from build123d import *

# Parameters (mm, degrees)
SKETCH1_W           = 19
SKETCH1_H           = 22
BOSS_EXTRUDE1_DEPTH = 22
SKETCH2_R           = 3.175
CUT_EXTRUDE1_DEPTH  = 22
SKETCH3_R           = 7.5
CUT_EXTRUDE2_DEPTH  = 5.5
SKETCH4_W           = 2
SKETCH4_H           = 3
CUT_EXTRUDE5_DEPTH  = 11


with BuildPart() as part:
    # Sketch1 → Boss-Extrude1 (new body)
    with BuildSketch(Plane(origin=(0, 0, 0), x_dir=(1, 0, 0), z_dir=(0, 1, 0))):
        Rectangle(SKETCH1_W, SKETCH1_H)
    extrude(amount=-BOSS_EXTRUDE1_DEPTH)

    # Sketch2 → Cut-Extrude1 (cut)
    with BuildSketch(Plane(origin=(0, 0, 0), x_dir=(1, 0, 0), z_dir=(0, 1, 0))):
        with Locations(Location((0, 0, 0), (0, 0, 270))):
            Circle(SKETCH2_R)
    extrude(amount=-CUT_EXTRUDE1_DEPTH, mode=Mode.SUBTRACT)

    # Sketch3 → Cut-Extrude2 (cut)
    with BuildSketch(Plane.XZ.offset(22)):
        with Locations(Location((0, 0, 0), (0, 0, 270))):
            Circle(SKETCH3_R)
    extrude(amount=-CUT_EXTRUDE2_DEPTH, mode=Mode.SUBTRACT)

    # Sketch4 → Cut-Extrude5 (cut)
    with BuildSketch(Plane(origin=(0, 0, 0), x_dir=(1, 0, 0), z_dir=(0, 1, 0))):
        with Locations((8.5, 0)):
            Rectangle(SKETCH4_W, SKETCH4_H)
    extrude(amount=-CUT_EXTRUDE5_DEPTH, mode=Mode.SUBTRACT)


solid = part.part
Source: CAD feature listing. Evaluate the final solid. Frame: model axes, mm. A direction names the side the tool comes from. Round coordinates to 2 decimals unless told otherwise and drop trailing zeros. Order: outer loops, then holes, each group sorted by start corner. A loop starts at its lowest first (then second) coordinate and runs counter-clockwise, first axis right, second up. Notation, with made-up numbers: (7, 74.5) - (49, 74.5) arc R27 ccw to (49, 108.5) - close; hole circle Ø9 at (28.25, 86). An arc over 180 degrees is marked (long way). Use a Markdown table: item, result. Add a question column.
1. Section query D-D (x = 6.75). Return the cut outline in (y, z), then the cut area to 3 significant figures.
2. Section query C-C (y = -5.75). Return the cut outline in (x, z) (3 decimals), then the cut area to 3 significant figures.
3. Section query A-A (x = 0). Return the cut outline in (y, z) (3 decimals), then the cut area to 3 significant figures.
4. Mould query, pull axis X, two halves, no side actions, for faces 4 (the flat face through (9.5, -13, 0)), 5 (the cylindrical face through (-1.93, -8.13, -2.52)), 6 (the cylindrical face through (0.33, -19.288, 7.493)), 7 (the flat face through (8, -11, 0)). Classes: +X half, -X half, draft (parallel to the pull), parting line (faces both ways), or undercut.
5. Set-up query: faces 1 (the flat face through (8, -5, 1.5)), 2 (the flat face through (0, -11, -11)), 3 (the flat face through (-2, -16.5, -3)). Return all of +Z, -Z, +X, -X, +Y, -Y with unobstructed straight access to the full face (end or side cutting, diameter ignored); none if empty.
6. First-contact query: pin 1 (6 mm diameter, centred on x = 3, z = 2, fed in from -Y). Flat tip, straight axial feed; report the tip coordinate or a pass-through.
7. Line query: probe 1 along X at (y, z) = (-19.15, 0); probe 2 along X at (y, z) = (-10.5, 0) (3 decimals); probe 3 along Y at (x, z) = (0, 4). Output: solid intervals per line, ascending.
8. Section query B-B (z = 0). Return the cut outline in (x, y) (3 decimals).
Derived:
| question | item | result |
|---|---|---|
| 1 | outline | (-22, -11) - (0, -11) - (0, 11) - (-22, 11) - (-22, 3.27) - (-16.5, 3.27) - (-16.5, -3.27) - (-22, -3.27) - close |
| 1 | area | 448 mm2 |
| 2 | outline | (-9.5, -11) - (9.5, -11) - (9.5, -1.5) - (7.5, -1.5) - (7.5, 1.5) - (9.5, 1.5) - (9.5, 11) - (-9.5, 11) - close; hole circle Ø6.35 at (0, 0) |
| 2 | area | 380 mm2 |
| 3 | outline | (-22, -11) - (0, -11) - (0, -3.175) - (-16.5, -3.175) - (-16.5, -7.5) - (-22, -7.5) - close; (-22, 7.5) - (-16.5, 7.5) - (-16.5, 3.175) - (0, 3.175) - (0, 11) - (-22, 11) - close |
| 3 | area | 297 mm2 |
| 4 | face 4 | +X half |
| 4 | face 5 | undercut |
| 4 | face 6 | undercut |
| 4 | face 7 | draft |
| 5 | face 1 | +X, +Y |
| 5 | face 2 | -Z, +X, -X, +Y, -Y |
| 5 | face 3 | -Y |
| 6 | pin 1 | y = -16.5 |
| 7 | probe 1 | -9.5 to -7.5, 7.5 to 9.5 |
| 7 | probe 2 | -9.5 to -3.175, 3.175 to 7.5 |
| 7 | probe 3 | -16.5 to 0 |
| 8 | outline | (-9.5, -22) - (-7.5, -22) - (-7.5, -16.5) - (-3.175, -16.5) - (-3.175, 0) - (-9.5, 0) - close; (3.175, -16.5) - (7.5, -16.5) - (7.5, -22) - (9.5, -22) - (9.5, -11) - (7.5, -11) - (7.5, 0) - (3.175, 0) - close |
